Answer from the drawing. Dimensions are ordinates in mm from the lowest x, y and z of the part. A direction names the side the tool comes from. Coordinates: 2 decimals unless noted, no trailing zeros. Loops run counter-clockwise (first coordinate to the right, second up) from the corner with the lowest first, then second, coordinate; pieces in that order, holes last. Notation, with made-up numbers: (51.25, -36.75) -> (75.25, -36.75) arc R34 cw to (75.25, -6.75) -> close; hole circle Ø7 at (84, 4.5). An arc over 180 degrees is marked (long way). Use a Markdown table: item, result.
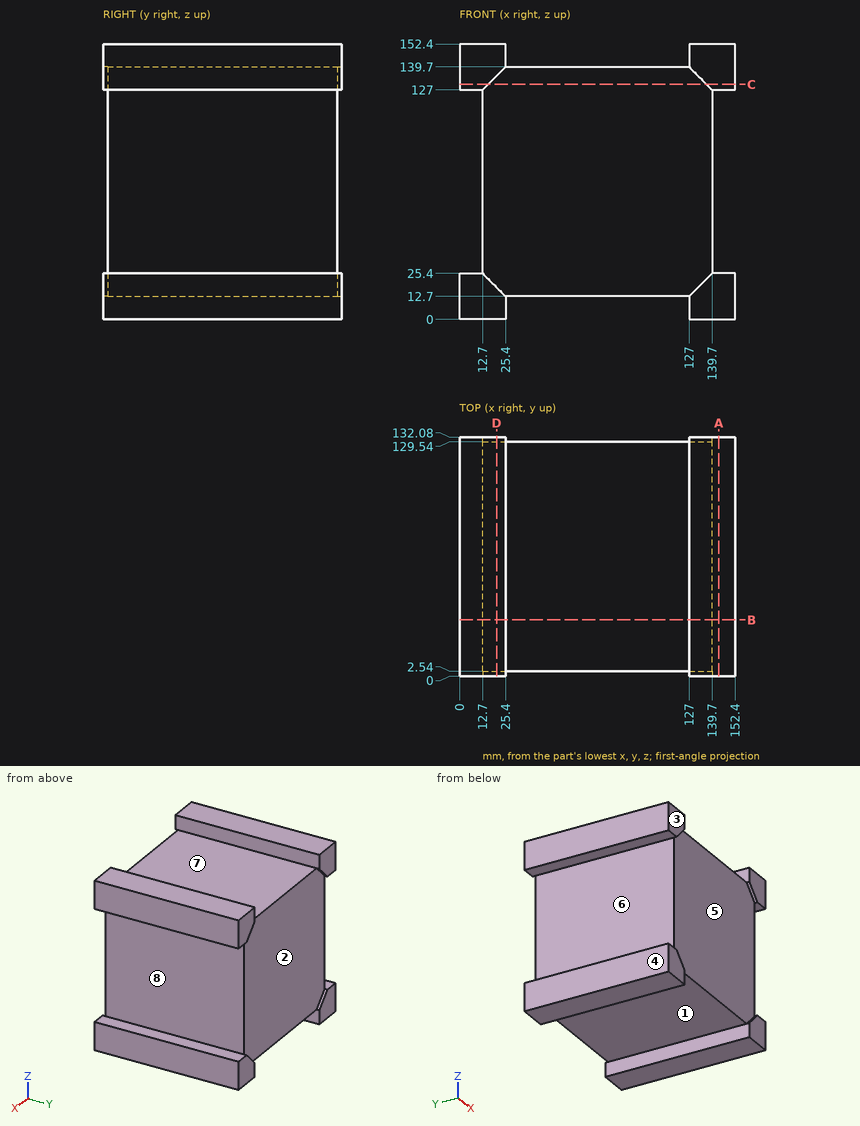
Q1. Section B-B on y = 31 is taken. Determine the outline of the cut face in (x, z), and give its area (3 significant figures).
Solved:
| item | result |
|---|---|
| outline | (0, 0) -> (25.4, 0) -> (25.4, 12.7) -> (127, 12.7) -> (127, 0) -> (152.4, 0) -> (152.4, 25.4) -> (139.7, 25.4) -> (139.7, 127) -> (152.4, 127) -> (152.4, 152.4) -> (127, 152.4) -> (127, 139.7) -> (25.4, 139.7) -> (25.4, 152.4) -> (0, 152.4) -> (0, 127) -> (12.7, 127) -> (12.7, 25.4) -> (0, 25.4) -> close |
| area | 18,100 mm² |
Q2. Section A-A on x = 143.5 is taken. Determine the outline of the cut face in (y, z).
Solved:
| item | result |
|---|---|
| outline | (0, 0) -> (132.08, 0) -> (132.08, 25.4) -> (0, 25.4) -> close; (0, 127) -> (132.08, 127) -> (132.08, 152.4) -> (0, 152.4) -> close |
Q3. Section C-C on z = 130 is taken. Determine the outline of the cut face in (x, y).
Solved:
| item | result |
|---|---|
| outline | (0, 0) -> (15.7, 0) -> (15.7, 2.54) -> (136.7, 2.54) -> (136.7, 0) -> (152.4, 0) -> (152.4, 132.08) -> (136.7, 132.08) -> (136.7, 129.54) -> (15.7, 129.54) -> (15.7, 132.08) -> (0, 132.08) -> close |
Q4. Determine the mould class of the marked faces 1, 2, 3 and 4 for opening direction X: pulls with the +X half, pulls with the -X half, needs draft (parallel to the pull), parting line crosses it, or undercut.
Solved:
| item | result |
|---|---|
| face 1 | undercut |
| face 2 | undercut |
| face 3 | needs draft |
| face 4 | pulls with the -X half |
Q5. Consider line 1 (Z direction, x = 6.5, y = 51); line 2 (X direction, y = 71.5, z = 33.5). Determine where each line is inside the solid, lowest interval first. Write a range as [from, to].
Solved:
| item | result |
|---|---|
| line 1 | [0, 25.4], [127, 152.4] |
| line 2 | [12.7, 139.7] |
Q6. For the marked faces 5, 6, 7 and 8, determine the directions among +Z, -Z, +X, -X, +Y, -Y from which every point of the face is accessible in a straight line to the end or side of a thin tool.
Solved:
| item | result |
|---|---|
| face 5 | -Y |
| face 6 | -X, +Y, -Y |
| face 7 | +Z, +Y, -Y |
| face 8 | +X, +Y, -Y |
Q7. Given pin 1 Ø4 at (y, z) = (54, 88) entering from +X; pin 2 Ø8 at (y, z) = (31.5, 37) entering from -X; pin 3 Ø10 at (x, z) = (72, 72) entering from -Y, each flat-ended and moving along its own axis, determine where each tip first touches the part or whether it passes through.
Solved:
| item | result |
|---|---|
| pin 1 | x = 139.7 |
| pin 2 | x = 12.7 |
| pin 3 | y = 2.54 |
Q8. Section D-D on x = 20.5 is taken. Determine the outline of the cut face in (y, z).
Solved:
| item | result |
|---|---|
| outline | (0, 0) -> (132.08, 0) -> (132.08, 17.6) -> (129.54, 17.6) -> (129.54, 134.8) -> (132.08, 134.8) -> (132.08, 152.4) -> (0, 152.4) -> (0, 134.8) -> (2.54, 134.8) -> (2.54, 17.6) -> (0, 17.6) -> close |
